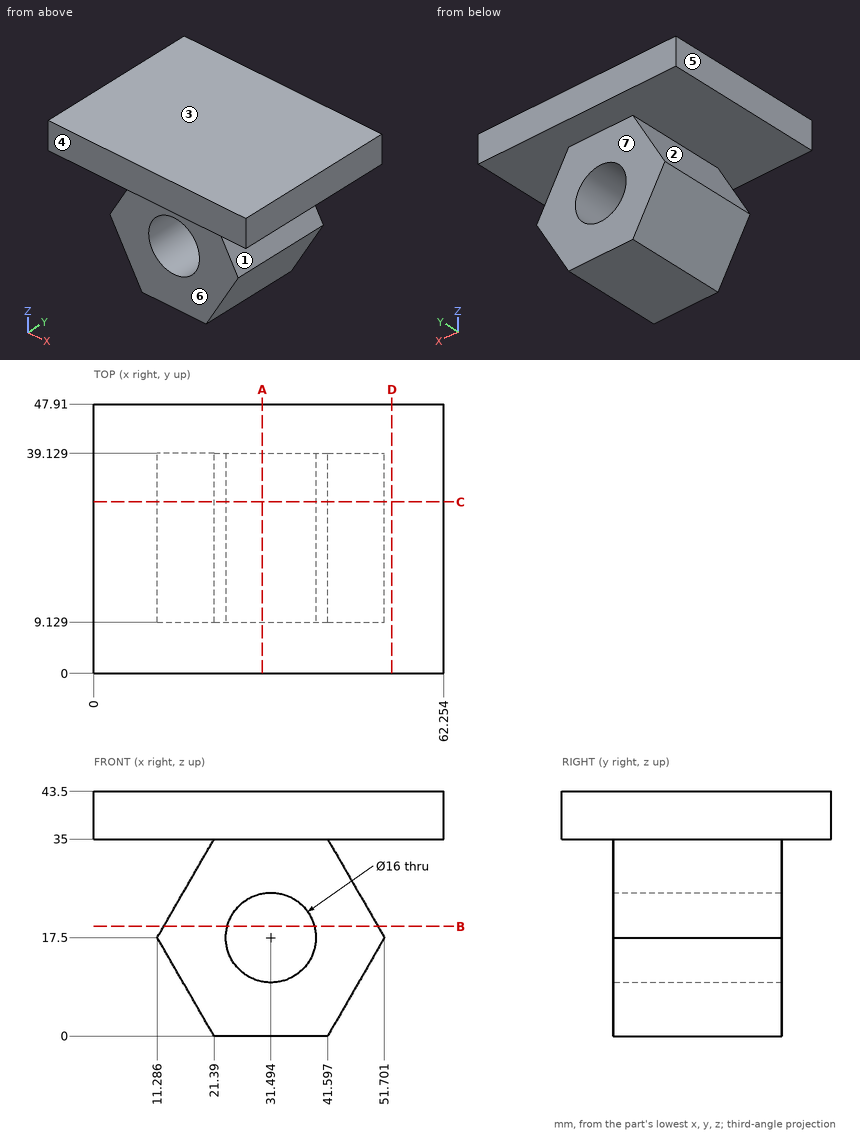
Design review of the part shown in the three views and the two pictorial views. Dimensions are in mm from the part's minimum x, y and z. A direction names the side the tool comes from. Give positions to 0.01 mm unless a question says otherwise; leave off trailing zeros. Order: outer loops, then holes, each group sorted by start corner. A loop starts at its lowest first (then second) coordinate and runs counter-clockwise, first axis right, second up. Notation, with made-up numbers: (-40, 5.5) -> (12, 5.5) arc R31 cw to (12, 34.5) -> close; hole circle Ø6 at (24.5, 79.25). An arc over 180 degrees is marked (long way). Write each question's results on one line, items separated by ' | '. Start each with the question number.
Q1. Add section B-B on z = 19.5. Give the boundary of the cut face in (x, y).
Q2. Add section A-A on x = 30. Give the boundary of the cut face in (y, z).
Q3. Add section C-C on y = 30.5. Give the boundary of the cut face in (x, z), and give its area (3 significant figures).
Q4. For pin 1 (12 mm diameter, centred on x = 10, z = 11, fed in from -Y); pin 2 (17.5 mm diameter, centred on x = 29.5, z = 19, fed in from +Y); pin 3 (4 mm diameter, centred on y = 16, z = 29.5, fed in from -X); pin 4 (14.5 mm diameter, centred on x = 31.49, z = 17.5, fed in from -Y), all flat-tipped, find the tip position at first contact; note any pin that passes through.
Q5. Mouldability with a two-part tool opening along Z and no side actions: class the marked faces 1, 2, 3 and 4 as +Z half, -Z half, draft (parallel to the pull), parting line (faces both ways), or undercut.
Q6. Machinability: for the marked faces 5, 6 and 7, which of the approach directions +Z, -Z, +X, -X, +Y, -Y give a long, thin tool a straight path to every point of the face, cutting with its end or side? Answer none if there is none.
Q7. Add section D-D on x = 53. Give the boundary of the cut face in (y, z).
Q8. Wall thickness on L1, parallel to Z at x = 31, y = 14.5 (1 decimal); L2, parallel to Y at x = 47, z = 20; L3, parallel to Z at x = 49, y = 16 (1 decimal): over which ranges is each line inside the solid? List them lowest first. Write a range as from..to.
Found:
1) outline: (12.44, 9.13) -> (23.75, 9.13) -> (23.75, 39.13) -> (12.44, 39.13) -> close; (39.24, 9.13) -> (50.55, 9.13) -> (50.55, 39.13) -> (39.24, 39.13) -> close
2) outline: (0, 35) -> (9.13, 35) -> (9.13, 25.36) -> (39.13, 25.36) -> (39.13, 35) -> (47.91, 35) -> (47.91, 43.5) -> (0, 43.5) -> close; (9.13, 0) -> (39.13, 0) -> (39.13, 9.64) -> (9.13, 9.64) -> close
3) outline: (0, 35) -> (21.39, 35) -> (11.29, 17.5) -> (21.39, 0) -> (41.6, 0) -> (51.7, 17.5) -> (41.6, 35) -> (62.25, 35) -> (62.25, 43.5) -> (0, 43.5) -> close; hole circle Ø16 at (31.49, 17.5) | area: 1,390 mm2
4) pin 1: stops at y = 9.13 | pin 2: stops at y = 39.13 | pin 3: stops at x = 17.06 | pin 4: passes through
5) face 1: undercut | face 2: undercut | face 3: +Z half | face 4: draft
6) face 5: +Z, -Z, -X, +Y, -Y | face 6: -Z, +X, -X, -Y | face 7: -Z, +X, -X, +Y
7) outline: (0, 35) -> (47.91, 35) -> (47.91, 43.5) -> (0, 43.5) -> close
8) L1: z = 0..9.5, 25.5..43.5 | L2: y = 9.13..39.13 | L3: z = 12.8..22.2, 35..43.5
